from build123d import *

# Parameters (mm, degrees)
F0_R            = 37.5
F1_DEPTH        = 45.4
F2_R            = 2
F3_DEPTH        = 45.401
F3_COPIES_COUNT = 6
F5_DEPTH        = 3.25
F5_COPIES_COUNT = 6
F7_DEPTH        = 8.4582
F8_W            = 76.2
F8_H            = 3.81
F9_DEPTH        = 8.4582
F11_R           = 4.064
F12_DEPTH       = 2.54
F13_R           = 4.7625
F14_DEPTH       = 36.9428001


# Not quite as in the source:
# - a pattern or mirror of a feature is missing from the dataset's text; its kind, count and spacing are read off the source's solid


with BuildPart() as f1:
    # F0 (on Front) → F1 (new body)
    with BuildSketch(Plane.XZ):
        Circle(F0_R)
    extrude(amount=F1_DEPTH)

    # F2 (on Front) → F3 (cut, through all)
    with BuildSketch(Plane.XZ):
        with Locations((0, 30)):
            Circle(F2_R)
    f3 = extrude(amount=F3_DEPTH, mode=Mode.SUBTRACT)

    # F3_copies: F3 ×6 about axis
    f3_copies_axis = Axis((0, 0, 0), (0, 1, 0))
    for i in range(1, F3_COPIES_COUNT):
        add(f3.rotate(f3_copies_axis, i * 360 / F3_COPIES_COUNT), mode=Mode.SUBTRACT)

    # F4 (on face) → F5 (cut)
    with BuildSketch(Plane.XZ.offset(45.4)):
        Polygon((2.3749, 34.1134474629), (-2.3749, 34.1134474629), (-4.7498, 30), (-2.3749, 25.8865525371), (2.3749, 25.8865525371), (4.7498, 30), align=None)
    f5 = extrude(amount=-F5_DEPTH, mode=Mode.SUBTRACT)

    # F5_copies: F5 ×6 about axis
    f5_copies_axis = Axis((0, 0, 0), (0, 1, 0))
    for i in range(1, F5_COPIES_COUNT):
        add(f5.rotate(f5_copies_axis, i * 360 / F5_COPIES_COUNT), mode=Mode.SUBTRACT)

    # F6 (on face) → F7 (cut)
    with BuildSketch(Plane(origin=(0, 0, 0), x_dir=(-1, 0, 0), z_dir=(0, 1, 0))):
        Polygon((-4.1574415534, -7.2009), (4.1574415534, -7.2009), (8.3148831068, 0), (4.1574415534, 7.2009), (-4.1574415534, 7.2009), (-8.3148831068, 0), align=None)
    extrude(amount=-F7_DEPTH, mode=Mode.SUBTRACT)

    # F8 (on face) → F9 (cut, through all)
    with BuildSketch(Plane(origin=(0, 0, 0), x_dir=(-1, 0, 0), z_dir=(0, 1, 0))):
        Rectangle(F8_W, F8_H)
    extrude(amount=-F9_DEPTH, mode=Mode.SUBTRACT)

    # F11 (on 3pt) → F12 (cut)
    with BuildSketch(Plane.YZ.offset(37.4515817423)):
        with Locations((-4.2291, 0)):
            Circle(F11_R)
    extrude(amount=-F12_DEPTH, mode=Mode.SUBTRACT)

    # F13 (on face) → F14 (cut, through all)
    with BuildSketch(Plane(origin=(0, -8.4582, 0), x_dir=(-1, 0, 0), z_dir=(0, 1, 0))):
        Circle(F13_R)
    extrude(amount=-F14_DEPTH, mode=Mode.SUBTRACT)


solid = f1.part
Could you check a few things on this model? Use its own coordinates, in mm. A direction names the side the tool comes from. Round coordinates to 2 decimals unless told otherwise and drop trailing zeros. Order: outer loops, then holes, each group sorted by start corner. A loop starts at its lowest first (then second) coordinate and runs counter-clockwise, first axis right, second up.
(1) Imagine slicing it at B-B (y = -21.5). Write out the boundary of the cut face in (x, z) (1 decimal).
Response values:
outline: circle Ø75 at (0, 0); hole circle Ø4 at (-26, -15); hole circle Ø4 at (-26, 15); hole circle Ø9.5 at (0, 0); hole circle Ø4 at (0, -30); hole circle Ø4 at (0, 30); hole circle Ø4 at (26, -15); hole circle Ø4 at (26, 15)
(2) I'm going to push flat-ended pins straight in: pin 1 (2.5 mm diameter, centred on x = -25, z = -15, fed in from -Y); pin 2 (4 mm diameter, centred on x = 25.5, y = -6, fed in from -Z); pin 3 (2.5 mm diameter, centred on x = 25.5, y = -44, fed in from +Z). Where does each tip first touch, or does it pass through?
Response values:
pin 1: stops at y = -42.15
pin 2: stops at z = -29.22
pin 3: stops at z = 28.6
(3) Imagine slicing it at C-C (z = -3). Write out the boundary of the cut face in (x, y), plus the area to 3 significant figures.
Response values:
outline: (-37.38, -45.4) - (-3.7, -45.4) - (-3.7, -8.46) - (-6.58, -8.46) - (-6.58, 0) - (-37.38, 0) - close; (3.7, -45.4) - (37.38, -45.4) - (37.38, -6.97) - (34.91, -6.97) - (34.91, -1.49) - (37.38, -1.49) - (37.38, 0) - (6.58, 0) - (6.58, -8.46) - (3.7, -8.46) - close
area: 3,000 mm2
(4) Imagine slicing it at A-A (x = 0). Write out the boundary of the cut face in (y, z).
Response values:
outline: (-45.4, -37.5) - (0, -37.5) - (0, -32) - (-42.15, -32) - (-42.15, -34.11) - (-45.4, -34.11) - close; (-45.4, -25.89) - (-42.15, -25.89) - (-42.15, -28) - (0, -28) - (0, -7.2) - (-8.46, -7.2) - (-8.46, -4.76) - (-45.4, -4.76) - close; (-45.4, 4.76) - (-8.46, 4.76) - (-8.46, 7.2) - (0, 7.2) - (0, 28) - (-42.15, 28) - (-42.15, 25.89) - (-45.4, 25.89) - close; (-45.4, 34.11) - (-42.15, 34.11) - (-42.15, 32) - (0, 32) - (0, 37.5) - (-45.4, 37.5) - close
(5) Please list where these lines run through material, in increasing order: line 1 along Z through (x, y) = (0, -20); line 2 along Z through (x, y) = (1.5, -36); line 3 along Z through (x, y) = (26, -16).
Response values:
line 1: z = -37.5 to -32, -28 to -4.76, 4.76 to 28, 32 to 37.5
line 2: z = -37.47 to -31.32, -28.68 to -4.52, 4.52 to 28.68, 31.32 to 37.47
line 3: z = -27.02 to -17, -13 to 13, 17 to 27.02
(6) If we mould it in two halves opening along Z, with no side actions, what happens to faces 1 (the cylindrical face through (-24.073, -20.78, -14.399)), 2 (the flat face through (-1, 0, 16)), 3 (the cylindrical face through (35.77, -22.38, 11.26))? For each: released by +Z, released by -Z, zero draft, split by the parting line, or undercut.
Response values:
face 1: undercut
face 2: zero draft
face 3: split by the parting line
(7) Imagine slicing it at D-D (x = -8.5). Write out the boundary of the cut face in (y, z) (3 decimals).
Response values:
outline: (-45.4, -36.524) - (0, -36.524) - (0, -1.905) - (-8.458, -1.905) - (-8.458, 1.905) - (0, 1.905) - (0, 36.524) - (-45.4, 36.524) - close
(8) Which directions (+Z, -Z, +X, -X, +Y, -Y) give clear straight access to the entire face, cutting with the end or side of a thin tool? Please do faces 4 (the flat face through (-22, -4, 1.905)), 5 (the flat face through (3, -8.458, 4)), 6 (the flat face through (29.526, -43.798, 12.914)), 7 (the cylindrical face through (36.199, -4.291, -4.064)).
Response values:
face 4: +X, -X, +Y
face 5: +Y
face 6: -Y
face 7: +X
